```python
from build123d import *

# Parameters (mm, degrees)
SKETCH_1_R      = 1.1
SKETCH_1_R_2    = 5.1
SKETCH_1_R_3    = 2.5
EXTRUDE_1_DEPTH = 2


with BuildPart() as part:
    # 草图1 → 凸台-拉伸1 (new body)
    with BuildSketch(Plane.XY):
        with BuildLine():
            Line((3.333333333, 9.428090416), (16.666666667, 4.714045208))
            ThreePointArc((16.666666667, 4.714045208), (20, 0), (16.666666667, -4.714045208))
            Line((16.666666667, -4.714045208), (3.333333333, -9.428090416))
            ThreePointArc((3.333333333, -9.428090416), (0, -10), (-3.333333333, -9.428090416))
            Line((-3.333333333, -9.428090416), (-16.666666667, -4.714045208))
            ThreePointArc((-16.666666667, -4.714045208), (-20, 0), (-16.666666667, 4.714045208))
            Line((-16.666666667, 4.714045208), (-3.333333333, 9.428090416))
            ThreePointArc((-3.333333333, 9.428090416), (0, 10), (3.333333333, 9.428090416))
        make_face()
        with Locations((0, 8)):
            Circle(SKETCH_1_R, mode=Mode.SUBTRACT)
        with Locations((8, 0)):
            Circle(SKETCH_1_R, mode=Mode.SUBTRACT)
        with Locations((0, -8)):
            Circle(SKETCH_1_R, mode=Mode.SUBTRACT)
        with Locations((-8, 0)):
            Circle(SKETCH_1_R, mode=Mode.SUBTRACT)
        Circle(SKETCH_1_R_2, mode=Mode.SUBTRACT)
        with Locations((15, 0)):
            Circle(SKETCH_1_R_3, mode=Mode.SUBTRACT)
        with Locations(Location((-15, 0, 0), (0, 0, 180))):
            Circle(SKETCH_1_R_3, mode=Mode.SUBTRACT)
    extrude(amount=EXTRUDE_1_DEPTH)


solid = part.part
```
Can you work these out from the model? Positions are in its coordinate system, mm. Round coordinates to 2 decimals unless told otherwise and drop trailing zeros. Loops run counter-clockwise (first coordinate to the right, second up) from the corner with the lowest first, then second, coordinate; pieces in that order, holes last. Notation, with made-up numbers: (5, -28.75) -> (43, -28.75) arc R8 ccw to (43, -18.75) -> close; hole circle Ø5 at (11.5, 38.25). An arc over 180 degrees is marked (long way). One line per item, written item: value. Start each with the question number.
1. If we section it at C-C, the plane z = 0.8: Write out the boundary of the cut face in (x, y), then the cut area to 3 significant figures.
2. If we section it at A-A, the plane x = 0: Write out the boundary of the cut face in (y, z).
3. If we mould it in two halves opening along X, with no side actions, what happens to faces 1 (the cylindrical face through (12.5, 0.1, 1)), 2 (the cylindrical face through (0, 10, 1)), 3 (the flat face through (10.09, -7.04, 0.99))? For each: pulls with the +X half, pulls with the -X half, needs draft (parallel to the pull), parting line crosses it, or undercut.
4. If we section it at D-D, the plane x = -15.5: Write out the boundary of the cut face in (y, z).
5. If we section it at B-B, the plane y = 0: Write out the boundary of the cut face in (x, z), then the cut area to 3 significant figures.
6. If I drill on probe 1 along Y at (x, z) = (0, 1.6); probe 2 along X at (y, z) = (1.5, 0.65); probe 3 along Y at (x, z) = (13, 1.1), over which ranges is the centre line in solid material (lowest first)?
Calculated:
1. outline: (-16.67, -4.71) -> (-3.33, -9.43) arc R10 ccw to (3.33, -9.43) -> (16.67, -4.71) arc R5 ccw to (16.67, 4.71) -> (3.33, 9.43) arc R10 ccw to (-3.33, 9.43) -> (-16.67, 4.71) arc R5 ccw to start; hole circle Ø5 at (-15, 0); hole circle Ø2.2 at (-8, 0); hole circle Ø10.2 at (0, 0); hole circle Ø2.2 at (0, -8); hole circle Ø2.2 at (0, 8); hole circle Ø2.2 at (8, 0); hole circle Ø5 at (15, 0)
1. area: 418 mm²
2. outline: (-10, 0) -> (-9.1, 0) -> (-9.1, 2) -> (-10, 2) -> close; (-6.9, 0) -> (-5.1, 0) -> (-5.1, 2) -> (-6.9, 2) -> close; (5.1, 0) -> (6.9, 0) -> (6.9, 2) -> (5.1, 2) -> close; (9.1, 0) -> (10, 0) -> (10, 2) -> (9.1, 2) -> close
3. face 1: undercut
3. face 2: parting line crosses it
3. face 3: pulls with the +X half
4. outline: (-5.13, 0) -> (-2.45, 0) -> (-2.45, 2) -> (-5.13, 2) -> close; (2.45, 0) -> (5.13, 0) -> (5.13, 2) -> (2.45, 2) -> close
5. outline: (-20, 0) -> (-17.5, 0) -> (-17.5, 2) -> (-20, 2) -> close; (-12.5, 0) -> (-9.1, 0) -> (-9.1, 2) -> (-12.5, 2) -> close; (-6.9, 0) -> (-5.1, 0) -> (-5.1, 2) -> (-6.9, 2) -> close; (5.1, 0) -> (6.9, 0) -> (6.9, 2) -> (5.1, 2) -> close; (9.1, 0) -> (12.5, 0) -> (12.5, 2) -> (9.1, 2) -> close; (17.5, 0) -> (20, 0) -> (20, 2) -> (17.5, 2) -> close
5. area: 30.8 mm²
6. probe 1: y = -10 to -9.1, -6.9 to -5.1, 5.1 to 6.9, 9.1 to 10
6. probe 2: x = -19.77 to -17, -13 to -4.87, 4.87 to 13, 17 to 19.77
6. probe 3: y = -6.01 to -1.5, 1.5 to 6.01
